```python
from build123d import *

# Parameters (mm, degrees)
F0_R     = 8.5
F1_DEPTH = 6


with BuildPart() as f1:
    # F0 (on Front) → F1 (new body)
    with BuildSketch(Plane.XZ):
        with BuildLine():
            ThreePointArc((12.5, 0), (9.897185, 7.635165), (3.172682, 12.090661))
            ThreePointArc((3.172682, 12.090661), (0.177882, 12.498734), (-2.827318, 12.176053))
            ThreePointArc((-2.827318, 12.176053), (-10.73528, 6.403418), (-12.057161, -3.297707))
            ThreePointArc((-12.057161, -3.297707), (-10.913162, -6.095317), (-9.131112, -8.536556))
            ThreePointArc((-9.131112, -8.536556), (-0.177882, -12.498734), (8.884479, -8.792954))
            ThreePointArc((8.884479, -8.792954), (10.73528, -6.403418), (11.95843, -3.639497))
            ThreePointArc((11.95843, -3.639497), (12.363866, -1.839785), (12.5, 0))
        make_face()
        Circle(F0_R, mode=Mode.SUBTRACT)
        with BuildLine():
            ThreePointArc((3.172682, 19.749459), (4.01393, 22.907963), (6.314776, 25.22959))
            ThreePointArc((6.314776, 25.22959), (-0.13188, 48.516555), (-6.085755, 25.098753))
            ThreePointArc((-6.085755, 25.098753), (-3.702196, 22.768604), (-2.827318, 19.552156))
            Line((-2.827318, 19.552156), (-2.827318, 12.176053))
            ThreePointArc((-2.827318, 12.176053), (0.177882, 12.498734), (3.172682, 12.090661))
            Line((3.172682, 12.090661), (3.172682, 19.749459))
        make_face()
        with Locations((0, 36.01725)):
            Circle(F0_R, mode=Mode.SUBTRACT)
        with BuildLine():
            ThreePointArc((-9.131112, -8.536556), (-10.913162, -6.095317), (-12.057161, -3.297707))
            Line((-12.057161, -3.297707), (-22.307375, -9.215671))
            ThreePointArc((-22.307375, -9.215671), (-41.927134, -24.412043), (-19.233423, -14.369128))
            Line((-19.233423, -14.369128), (-9.131112, -8.536556))
        make_face()
        with Locations((-31.191854, -18.008625)):
            Circle(F0_R, mode=Mode.SUBTRACT)
        with BuildLine():
            Line((22.060741, -9.472069), (11.95843, -3.639497))
            ThreePointArc((11.95843, -3.639497), (10.73528, -6.403418), (8.884479, -8.792954))
            Line((8.884479, -8.792954), (19.134693, -14.710918))
            ThreePointArc((19.134693, -14.710918), (42.105016, -24.103942), (22.060741, -9.472069))
        make_face()
        with Locations((31.191854, -18.008625)):
            Circle(F0_R, mode=Mode.SUBTRACT)
    extrude(amount=F1_DEPTH)


solid = f1.part
```
Work out the finished part from the listing and answer in its coordinate system (mm). A direction names the side the tool comes from. Give positions to 0.01 mm unless a question says otherwise; leave off trailing zeros. Loops run counter-clockwise (first coordinate to the right, second up) from the corner with the lowest first, then second, coordinate; pieces in that order, holes last. Notation, with made-up numbers: (49, -0.5) -> (60, -0.5) arc R11 ccw to (60, 15.5) -> close; hole circle Ø6 at (70, -17). An arc over 180 degrees is marked (long way). Write item = value, one per line. Start each with the question number.
(1) Which of the six approach directions +Z, -Z, +X, -X, +Y, -Y give full straight-line access (tool end or side, diameter ignored) to faces 5 (the cylindrical face through (-1.84, -2.96, 27.72)), 6 (the flat face through (-2.827, -3, 16)), 7 (the flat face through (3.173, -3, 16))?
(2) Given pin 1 Ø1.5 at (y, z) = (-4.5, -14.5) entering from +X; pin 2 Ø2 at (x, y) = (23, -2.5) entering from -Z; pin 3 Ø3 at (y, z) = (-2, 16) entering from +X; pin 4 Ø19.5 at (x, z) = (0, 36.02) entering from -Y, each flat-ended and moving along its own axis, determine where each tip first touches the part or whether it passes through.
(3) Find section D-D on y = -3.2. Give the vertices of the cut face in (x, z).
(4) Find section C-C on x = 25. Give the vertices of the cut face in (y, z).
(5) Find section A-A on z = 40.5. Give the vertices of the cut face in (x, y), and give its area (3 significant figures).
(6) Find section B-B on x = 0. Give the vertices of the cut face in (y, z).
(7) Find the intervals of material crossed by probe 1 along Z at (x, y) = (0, -2.05); probe 2 along X at (y, z) = (-0.6, -13.5); probe 3 along X at (y, z) = (-2.1, -14), in increasing order. Write a range as from..to.
(8) The mould has two halves that part along Z. Classify faces 1 (the flat face through (-3.4, 0, -8.4)), 2 (the cylindrical face through (39.3, -2.96, -15.46)), 3 (the cylindrical face through (-0.319, -2.958, -12.496)), 4 (the cylindrical face through (-23.084, -2.958, -15.455)): +Z half, -Z half, draft (parallel to the pull), parting line (faces both ways), or undercut.
From the geometry:
q1.face_5 = +Y, -Y
q1.face_6 = -X, +Y, -Y
q1.face_7 = +X, +Y, -Y
q2.pin_1 = 43.38
q2.pin_2 = -28.23
q2.pin_3 = 3.17
q2.pin_4 = -6
q3.outline = (-22.31, -9.22) arc R12.5 ccw (long way) to (-19.23, -14.37) -> (-9.13, -8.54) arc R12.5 ccw to (8.88, -8.79) -> (19.13, -14.71) arc R12.5 ccw (long way) to (22.06, -9.47) -> (11.96, -3.64) arc R12.5 ccw to (12.5, 0) arc R12.5 ccw to (3.17, 12.09) -> (3.17, 19.75) arc R6.35 cw to (6.31, 25.23) arc R12.5 ccw (long way) to (-6.09, 25.1) arc R6.35 cw to (-2.83, 19.55) -> (-2.83, 12.18) arc R12.5 ccw to (-12.06, -3.3) -> close; hole circle Ø17 at (-31.19, -18.01); hole circle Ø17 at (0, 0); hole circle Ø17 at (0, 36.02); hole circle Ø17 at (31.19, -18.01)
q4.outline = (-6, -28.87) -> (0, -28.87) -> (0, -23.83) -> (-6, -23.83) -> close; (-6, -12.19) -> (0, -12.19) -> (0, -7.15) -> (-6, -7.15) -> close
q5.outline = (-11.67, -6) -> (-7.22, -6) -> (-7.22, 0) -> (-11.67, 0) -> close; (7.22, -6) -> (11.67, -6) -> (11.67, 0) -> (7.22, 0) -> close
q5.area = 53.4 mm^2
q6.outline = (-6, -12.5) -> (0, -12.5) -> (0, -8.5) -> (-6, -8.5) -> close; (-6, 8.5) -> (0, 8.5) -> (0, 27.52) -> (-6, 27.52) -> close; (-6, 44.52) -> (0, 44.52) -> (0, 48.52) -> (-6, 48.52) -> close
q7.probe_1 = -12.5..-8.5, 8.5..27.52, 44.52..48.52
q7.probe_2 = -42.85..-38.4, -23.99..-17.73, 17.04..23.99, 38.4..42.85
q7.probe_3 = -43.03..-38.69, -23.7..-18.59, 17.9..23.7, 38.69..43.03
q8.face_1 = draft
q8.face_2 = undercut
q8.face_3 = -Z half
q8.face_4 = undercut
